from build123d import *

# Parameters (mm, degrees)
F3_D     = 17.5
F3_DEPTH = 32
F3_TIP   = 5.2575304165
F5_D     = 17.5
F5_DEPTH = 32
F5_TIP   = 5.2575304165


with BuildPart() as f1:
    # F0 (on Front) → F1 (revolve)
    with BuildSketch(Plane.XZ):
        with BuildLine():
            Line((0, 77.5), (0, 0))
            Line((0, 0), (170, 0))
            Line((170, 0), (170, 40.304846024))
            ThreePointArc((170, 40.304846024), (169.5867066806, 41.5223688821), (168.5176380902, 42.2366976766))
            Line((168.5176380902, 42.2366976766), (164.75, 43.2462332603))
            Line((164.75, 43.2462332603), (164.75, 41.8395))
            Line((164.75, 41.8395), (158.25, 41.8395))
            Line((158.25, 41.8395), (158.25, 44.9879030111))
            Line((158.25, 44.9879030111), (150.7407518075, 47))
            Line((150.7407518075, 47), (51, 47))
            ThreePointArc((51, 47), (50.2928932188, 47.2928932188), (50, 48))
            Line((50, 48), (50, 68.7798354631))
            ThreePointArc((50, 68.7798354631), (49.5867066806, 69.9973583211), (48.5176380902, 70.7116871157))
            Line((48.5176380902, 70.7116871157), (41.4, 72.6188524939))
            Line((41.4, 72.6188524939), (41.4, 66.4565))
            Line((41.4, 66.4565), (32.6, 66.4565))
            Line((32.6, 66.4565), (32.6, 74.9768053873))
            Line((32.6, 74.9768053873), (23.1833095082, 77.5))
            Line((23.1833095082, 77.5), (0, 77.5))
        make_face()
    revolve(axis=Axis((85, 0, 0), (1, 0, 0)))

    # F3
    with Locations(Plane(origin=(0, 0, 0), x_dir=(0, -1, 0), z_dir=(-1, 0, 0))):
        with Locations((0, 0)):
            Hole(F3_D / 2, depth=F3_DEPTH)
            with Locations((0, 0, -(F3_DEPTH + F3_TIP / 2))):  # 118° drill point
                Cone(0, F3_D / 2, F3_TIP, mode=Mode.SUBTRACT)

    # F5
    with Locations(Plane.YZ.offset(170)):
        with Locations((0, 0)):
            Hole(F5_D / 2, depth=F5_DEPTH)
            with Locations((0, 0, -(F5_DEPTH + F5_TIP / 2))):  # 118° drill point
                Cone(0, F5_D / 2, F5_TIP, mode=Mode.SUBTRACT)


solid = f1.part
Geometry check sheet. Reference: the model listing, model coordinates, mm. A direction names the side the tool comes from. Round coordinates to 2 decimals unless told otherwise and drop trailing zeros. Loops run counter-clockwise (first coordinate to the right, second up) from the corner with the lowest first, then second, coordinate; pieces in that order, holes last. Notation, with made-up numbers: (57, 0.5) -> (104, 0.5) arc R11 cw to (104, 11.5) -> close; hole circle Ø7 at (39.5, 88.5). An arc over 180 degrees is marked (long way). Answer as a JSON object with one key per item and string values. Group by question number.
Item 1: Thickness scan on line 1 along Z through (x, y) = (150, 0); line 2 along Z through (x, y) = (20, 0). Record the ranges inside material, lowest first.
Item 2: Depth check by flat-ended pin: pin 1 Ø16 at (y, z) = (0, 0) entering from +X; pin 2 Ø3 at (y, z) = (39, 47) entering from +X; pin 3 Ø12 at (x, z) = (136, -46) entering from -Y. Enter the tip coordinate at first touch or a pass-through.
Item 3: Release check for a two-part mould opening along Z. For faces 4 (the face through (50, 14, 47)), 5 (the face through (16.224, -6.944, -5.324)), 6 (the face through (48.07, -21.28, 67.56)) record: pulls with the +Z half, pulls with the -Z half, needs draft (parallel to the pull), parting line crosses it, or undercut.
Item 4: Set-up check for faces 1 (the face through (161.454, -41.483, -5.447)), 2 (the face through (170, -10, 1)), 3 (the face through (153.776, 6.944, -5.324)): record each of +Z, -Z, +X, -X, +Y, -Y from which the full face is reachable in a straight line by a thin tool's end or side.
Item 5: Cross-section at A-A, the plane x = 94. Record the cut outline in (y, z), plus the area to 3 significant figures.
Determined:
{
 "1": {"line 1": "z = -47 to -8.75, 8.75 to 47", "line 2": "z = -77.5 to -8.75, 8.75 to 77.5"},
 "2": {"pin 1": "stops at x = 137.55", "pin 2": "stops at x = 50", "pin 3": "stops at y = -24.68"},
 "3": {"face 4": "needs draft", "face 5": "undercut", "face 6": "parting line crosses it"},
 "4": {"face 1": "none", "face 2": "+Z, -Z, +X, +Y, -Y", "face 3": "+X"},
 "5": {"outline": "circle Ø94 at (0, 0)", "area": "6,940 mm²"}
}
